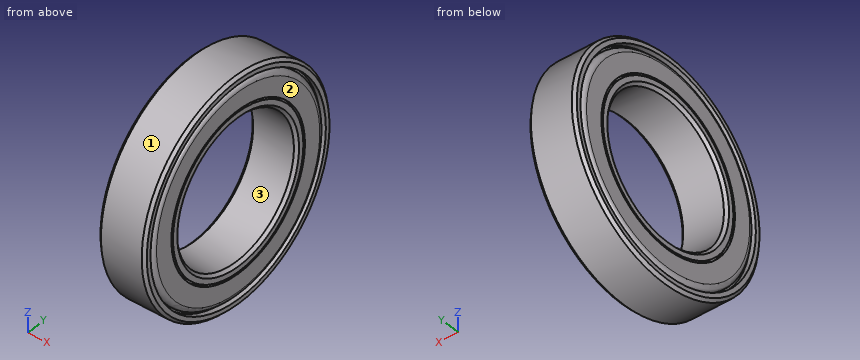
```python
from build123d import *

# Parameters (mm, degrees)
SKETCH1_R           = 12
SKETCH1_R_2         = 7.5
BOSS_EXTRUDE1_DEPTH = 2.5
CHAMFER1_SIZE       = 0.3


with BuildPart() as part:
    # Sketch1 → Boss-Extrude1 (new, symmetric)
    with BuildSketch(Plane(origin=(0, 0, 0), x_dir=(0, 0, -1), z_dir=(1, 0, 0))):
        Circle(SKETCH1_R)
        Circle(SKETCH1_R_2, mode=Mode.SUBTRACT)
    extrude(amount=BOSS_EXTRUDE1_DEPTH, both=True)

    # Chamfer1
    chamfer1_edges = [part.edges().sort_by_distance(p)[0] for p in [
        (-2.5, 0, 12),
        (2.5, 0, 12),
        (-2.5, 0, 7.5),
        (2.5, 0, 7.5),
    ]]
    chamfer(chamfer1_edges, length=CHAMFER1_SIZE)

    # Sketch2 → Cut-Revolve1 (revolve, cut)
    with BuildSketch(Plane.XY, mode=Mode.PRIVATE) as cut_revolve1_sk:
        with BuildLine():
            Line((2.93973246, 11.230084286), (1.92076619, 11.230084286))
            Line((1.92076619, 11.230084286), (1.92076619, 11.030084286))
            ThreePointArc((1.92076619, 11.030084286), (2.330346345, 10.860430631), (2.5, 10.450850477))
            Line((2.5, 10.450850477), (2.5, 8.554548016))
            Line((2.5, 8.554548016), (2.084848677, 8.554548016))
            Line((2.084848677, 8.554548016), (2.084848677, 8.354548016))
            Line((2.084848677, 8.354548016), (2.93973246, 8.354548016))
            Line((2.93973246, 8.354548016), (2.93973246, 11.230084286))
        make_face()
    cut_revolve1 = revolve(cut_revolve1_sk.sketch.rotate(Axis((3.211719083, 0, 0), (-1, 0, 0)), 90), axis=Axis((3.211719083, 0, 0), (-1, 0, 0)), mode=Mode.SUBTRACT)

    # Mirror1: Cut-Revolve1 across plane
    add(cut_revolve1.mirror(Plane(origin=(0, 0, 0), x_dir=(0, 0, 1), z_dir=(1, 0, 0))), mode=Mode.SUBTRACT)


solid = part.part
```
The model under review builds one solid part; all positions refer to its coordinate system, in mm. Face numbers are marked on the shaded views. Round coordinates to 2 decimals unless told otherwise and drop trailing zeros. Loops run counter-clockwise (first coordinate to the right, second up) from the corner with the lowest first, then second, coordinate; pieces in that order, holes last.
Item 1: Take a section at A-A (x = 1.2). Write out the cut boundary in (y, z), then the cut area to 3 significant figures.
Determined:
outline: circle Ø24 at (0, 0); hole circle Ø15 at (0, 0)
area: 276 mm2
Item 2: For line 1 (Y direction, x = -2.25, z = 0); line 2 (Z direction, x = 2, y = 1.25); line 3 (Y direction, x = -2.4, z = 0), list the stretches that pass through material, from the lowest coordinate up.
Determined:
line 1: y = -11.95 to -11.23, -10.93 to -8.55, -8.35 to -7.55, 7.55 to 8.35, 8.55 to 10.93, 11.23 to 11.95
line 2: z = -11.93 to -11.16, -10.95 to -7.4, 7.4 to 10.95, 11.16 to 11.93
line 3: y = -11.8 to -11.23, -10.78 to -8.55, -8.35 to -7.7, 7.7 to 8.35, 8.55 to 10.78, 11.23 to 11.8
Item 3: Mouldability with a two-part tool opening along Y and no side actions: class the marked faces 1, 2 and 3 as released by +Y, released by -Y, zero draft, split by the parting line, or undercut.
Determined:
face 1: split by the parting line
face 2: zero draft
face 3: undercut
Item 4: Clearance check with flat-ended pins moving along their axes: pin 1 Ø3 at (x, z) = (2, 2.5) entering from +Y; pin 2 Ø8.5 at (y, z) = (-2, -1) entering from +X; pin 3 Ø2 at (x, z) = (0, -7) entering from +Y; pin 4 Ø1 at (x, y) = (-1.5, -9.5) entering from -Z. State where each tip first meets the part, or that it passes through.
Determined:
pin 1: stops at y = 11.96
pin 2: passes through
pin 3: stops at y = 10.39
pin 4: stops at z = -7.94
